Can you work these out from the model? Positions are in its coordinate system, mm. A direction names the side the tool comes from. Give positions to 0.01 mm unless a question says otherwise; leave off trailing zeros. Order: outer loops, then holes, each group sorted by start corner. A loop starts at its lowest first (then second) coordinate and runs counter-clockwise, first axis right, second up. Notation, with made-up numbers: M 59.5,-20 L 80.5,-20 A34 ccw 80.5,16 Z; hole C 32.25,66.25 d5. An arc over 180 degrees is marked long. One line per question, with ' | ' between items. Start each with the question number.
1) If we section it at C-C, the plane x = 2.75: Please give me the cut outline in (y, z) (1 decimal), plus the area to 3 significant figures.
2) If we section it at A-A, the plane y = -13.5: Please give me the cut outline in (x, z).
3) I'm going to push a flat-ended pin straight in: pin 1 Ø4 at (x, z) = (6.5, 5.5) entering from -Y (3 decimals). Where does the tip first touch, or does it pass through?
4) If we section it at B-B, the plane z = 0: Please give me the cut outline in (x, y) (3 decimals), plus the area to 3 significant figures.
5) Thinking about a two-plate mould opening in Z: for faces 4 (the cylindrical face through (-1.1, -22.1, -12.7)), 5 (the flat face through (-2, -13, -14.288)), 6 (the flat face through (-1, -13, 14.56)), 7 (the cylindrical face through (-6.93, -1.57, -5.31)), which applies, +Z half, -Z half, draft (parallel to the pull), parting line (faces both ways), or undercut?
6) For faces 1 (the flat face through (-2, -25.4, -13)), 2 (the flat face through (-10, -3.175, 0)), 3 (the flat face through (0, -2, 11.112)), which set-ups out of +Z, -Z, +X, -X, +Y, -Y let a thin tool reach every point of the face, with its end or its side?
7) Please list where these lines run through material, in increasing order: line 1 along Z through (x, y) = (6.5, -7.5); line 2 along Z through (x, y) = (0, -2); line 3 along Y through (x, z) = (-9, -9.5) (3 decimals). Write a range as [from, to].
8) If we section it at D-D, the plane y = -17.25: Please give me the cut outline in (x, z).
```python
from build123d import *

# Parameters (mm, degrees)
F0_W     = 20.6375
F0_H     = 22.225
F0_R     = 8.73125
F1_DEPTH = 3.175
F2_DEPTH = 25.4
F4_D     = 7.14375


# Not quite as in the source:
# - a length typed as a fraction of an inch, garbled in the dataset ("3 / 203.2 mm" for 3/8 in), is restored


with BuildPart() as f1:
    # F0 (on Front) → F1 (new body)
    with BuildSketch(Plane.XZ):
        Rectangle(F0_W, F0_H)
        Circle(F0_R, mode=Mode.SUBTRACT)
        Polygon((-10.31875, -11.1125), (-10.31875, 11.1125), (-10.31875, 11.3854380324), (-13.49375, 11.3854380324), (-13.49375, -11.1125), align=None)
    extrude(amount=F1_DEPTH)

    # F0 (on Front) → F2 (join)
    with BuildSketch(Plane.XZ):
        Polygon((10.31875, -14.2875), (10.31875, -11.1125), (-10.31875, -11.1125), (-13.49375, -11.1125), (-13.49375, -14.2875), align=None)
        Polygon((-13.49375, 11.3854380324), (-10.31875, 11.3854380324), (10.31875, 11.3854380324), (10.31875, 14.5604380324), (-13.49375, 14.5604380324), align=None)
    extrude(amount=F2_DEPTH)

    # F4 (through all)
    with Locations(Plane(origin=(0, 0, -14.2875), x_dir=(1, 0, 0), z_dir=(0, 0, -1))):
        with Locations((-1.5875, 18.5598246753)):
            Hole(F4_D / 2)


solid = f1.part
```
Results found:
1) outline: M -25.4,-14.3 L 0,-14.3 L 0,-8.3 L -3.2,-8.3 L -3.2,-11.1 L -25.4,-11.1 Z; M -25.4,11.4 L 0,11.4 L 0,14.6 L -25.4,14.6 Z; M -3.2,8.3 L 0,8.3 L 0,11.1 L -3.2,11.1 Z | area: 179 mm²
2) outline: M -13.49,-14.29 L 10.32,-14.29 L 10.32,-11.11 L -13.49,-11.11 Z; M -13.49,11.39 L 10.32,11.39 L 10.32,14.56 L -13.49,14.56 Z
3) pin 1: stops at y = -3.175
4) outline: M -13.494,-3.175 L -8.731,-3.175 L -8.731,0 L -13.494,0 Z; M 8.731,-3.175 L 10.319,-3.175 L 10.319,0 L 8.731,0 Z | area: 20.2 mm²
5) face 4: draft | face 5: -Z half | face 6: +Z half | face 7: undercut
6) face 1: +Z, -Z, +X, -X, -Y | face 2: +X, -X, -Y | face 3: +X, +Y, -Y
7) line 1: z = [-14.29, -11.11], [11.39, 14.56] | line 2: z = [-14.29, -8.73], [8.73, 11.11], [11.39, 14.56] | line 3: y = [-3.175, 0]
8) outline: M -13.49,-14.29 L -4.91,-14.29 L -4.91,-11.11 L -13.49,-11.11 Z; M -13.49,11.39 L -4.91,11.39 L -4.91,14.56 L -13.49,14.56 Z; M 1.74,-14.29 L 10.32,-14.29 L 10.32,-11.11 L 1.74,-11.11 Z; M 1.74,11.39 L 10.32,11.39 L 10.32,14.56 L 1.74,14.56 Z
